Read the model definition and answer for the solid it produces. Units are mm, in the model's axes. Face numbers are marked on the shaded views. Coordinates: 2 decimals unless noted, no trailing zeros. Write each loop counter-clockwise with the first axis right and the second up, starting at its lowest first coordinate (ties: lowest second). Pieces come first, ordered by that corner, then holes. Notation, with made-up numbers: (74, 4) -> (129, 4) arc R10 ccw to (129, 11) -> close; hole circle Ø5 at (74.5, 28). An arc over 180 degrees is marked (long way). One line per item, written item: value. Start each with the question number.
1. Find section A-A, the plane x = -11. Write down the section's boundary in (y, z).
2. Find section B-B, the plane y = 0. Write down the section's boundary in (x, z).
3. Consider line 1 along Y through (x, z) = (-11, 1.25); line 2 along X through (y, z) = (4.75, 1.15); line 3 along X through (y, z) = (5.5, 2.05). Determine where each line is inside the solid, lowest interval first.
4. Find section C-C, the plane z = 2.55. Write down the section's boundary in (x, y).
5. For a pull along Y with two mould halves and no side action, classify the marked faces 1, 2 and 3 as pulls with the +Y half, pulls with the -Y half, needs draft (parallel to the pull), parting line crosses it, or undercut.
Autodesk Fusion 360 part; units mm, degrees
sketch "Sketch1" plane through (0, 0, 0) normal (0, 0, 1) x (1, 0, 0)
  line L0 (18, -6.5) -> (-18, -6.5)
  line L1 (-20, -4.5) -> (-20, 4.5)
  line L2 (-18, 6.5) -> (18, 6.5)
  line L3 (20, 4.5) -> (20, -4.5)
  line L4 (20, -6.5) -> (-20, 6.5) construction
  line L5 (-20, -6.5) -> (20, 6.5) construction
  arc A0 (20, 4.5) -> (18, 6.5) centre (18, 4.5) ccw
  arc A1 (18, -6.5) -> (20, -4.5) centre (18, -4.5) ccw
  arc A2 (-20, -4.5) -> (-18, -6.5) centre (-18, -4.5) ccw
  arc A3 (-18, 6.5) -> (-20, 4.5) centre (-18, 4.5) ccw
  line L6 (0, 0) -> (11, 0)
  line L7 (0, 0) -> (-11, 0) construction
  circle A4 centre (11, 0) radius 3
  circle A5 centre (-11, 0) radius 3
  dimension "d1" = 40
  dimension "d2" = 13
  dimension "d3" = 2
  dimension "d4" = 11
  dimension "d5" = 11
  dimension "d6" = 6
  dimension "d7" = 6
extrude "Extrude1" add sketch "Sketch1" along normal blind 3
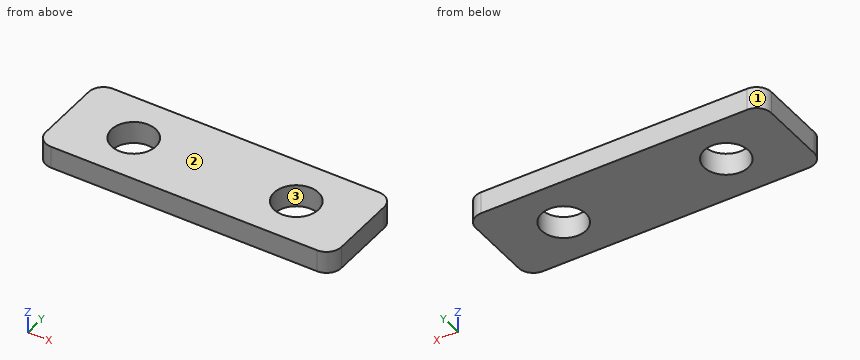
Answer block:
1. outline: (-6.5, 0) -> (-3, 0) -> (-3, 3) -> (-6.5, 3) -> close; (3, 0) -> (6.5, 0) -> (6.5, 3) -> (3, 3) -> close
2. outline: (-20, 0) -> (-14, 0) -> (-14, 3) -> (-20, 3) -> close; (-8, 0) -> (8, 0) -> (8, 3) -> (-8, 3) -> close; (14, 0) -> (20, 0) -> (20, 3) -> (14, 3) -> close
3. line 1: y = -6.5 to -3, 3 to 6.5
3. line 2: x = -19.98 to 19.98
3. line 3: x = -19.73 to 19.73
4. outline: (-20, -4.5) arc R2 ccw to (-18, -6.5) -> (18, -6.5) arc R2 ccw to (20, -4.5) -> (20, 4.5) arc R2 ccw to (18, 6.5) -> (-18, 6.5) arc R2 ccw to (-20, 4.5) -> close; hole circle Ø6 at (-11, 0); hole circle Ø6 at (11, 0)
5. face 1: pulls with the +Y half
5. face 2: needs draft
5. face 3: undercut
